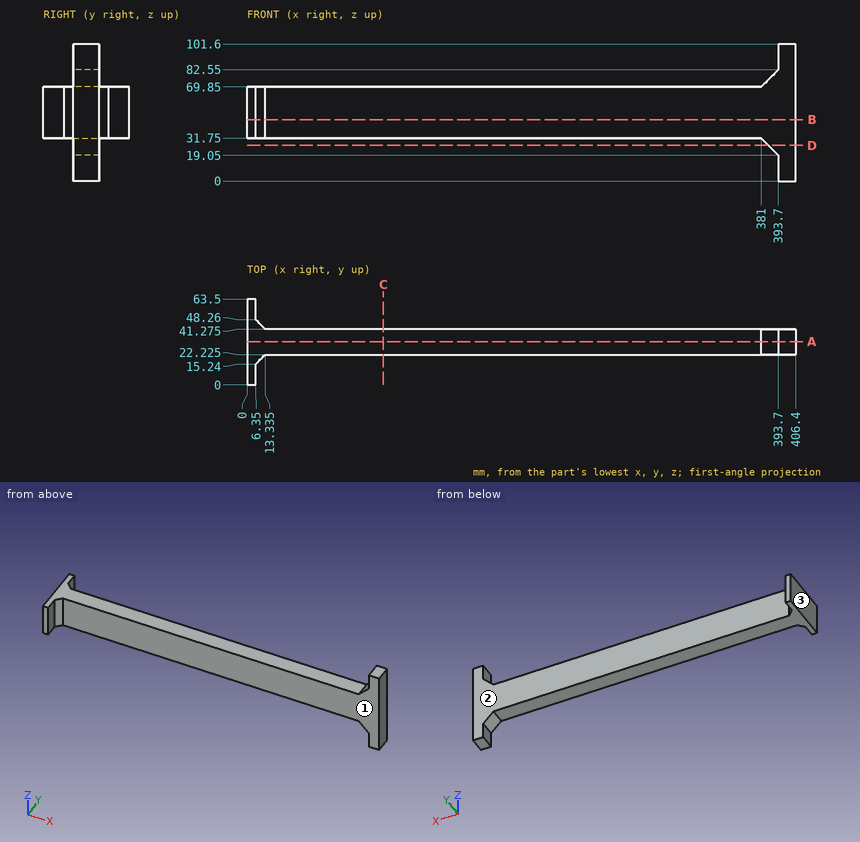
Study the drawing (mm; zero at the part's minimum x, y, z) and answer. A direction names the side the tool comes from. Give positions to 0.01 mm unless a question says otherwise; leave off trailing zeros. Loops run counter-clockwise (first coordinate to the right, second up) from the corner with the lowest first, then second, coordinate; pieces in that order, holes last. Notation, with made-up numbers: (-35.75, 74) - (5.25, 74) arc R28 cw to (5.25, 109) - close; hole circle Ø8 at (-6.75, 5). An arc over 180 degrees is marked (long way). Answer as CSV lines item,"result". Start each with the question number.
1) Find section B-B (z = 45.5). Write down the section's boundary in (x, y) (3 decimals).
2) Find section A-A (y = 32). Write down the section's boundary in (x, z).
3) Find section C-C (x = 101). Write down the section's boundary in (y, z) (3 decimals), then the cut area to 3 significant figures.
4) Each of these flat-tipped pins is pushed along its axis until it touches: pin 1 Ø19 at (x, y) = (133.5, 43) entering from +Z; pin 2 Ø19 at (x, y) = (180.5, 31) entering from -Z; pin 3 Ø12 at (y, z) = (8, 48) entering from +X. Where does it stop, or does it pass through?
5) Find section D-D (z = 26.5). Write down the section's boundary in (x, y) (3 decimals).
6) Straight lines are drawn through the part: L1, parallel to X at y = 12, z = 68; L2, parallel to Z at x = 281.5, y = 39.5; L3, parallel to Y at x = 358, z = 50 (3 decimals). For each, find the intervals that lie inside material, in ascending order. Write a range as from..to.
7) Which of the six approach directions +Z, -Z, +X, -X, +Y, -Y give full straight-line access (tool end or side, diameter ignored) to the marked faces 1, 2 and 3?
Findings below:
1,outline,"(0, 0) - (6.35, 0) - (6.35, 15.24) - (13.335, 22.225) - (406.4, 22.225) - (406.4, 41.275) - (13.335, 41.275) - (6.35, 48.26) - (6.35, 63.5) - (0, 63.5) - close"
2,outline,"(0, 31.75) - (381, 31.75) - (393.7, 19.05) - (393.7, 0) - (406.4, 0) - (406.4, 101.6) - (393.7, 101.6) - (393.7, 82.55) - (381, 69.85) - (0, 69.85) - close"
3,outline,"(22.225, 31.75) - (41.275, 31.75) - (41.275, 69.85) - (22.225, 69.85) - close"
3,area,"726 mm^2"
4,pin 1,"z = 69.85"
4,pin 2,"z = 31.75"
4,pin 3,"x = 6.35"
5,outline,"(386.25, 22.225) - (406.4, 22.225) - (406.4, 41.275) - (386.25, 41.275) - close"
6,L1,"0..6.35"
6,L2,"31.75..69.85"
6,L3,"22.225..41.275"
7,face 1,"+Z, -Z, +X, -Y"
7,face 2,"+Z, -Z, +X, +Y"
7,face 3,"+Z, -Z, -X, +Y, -Y"
